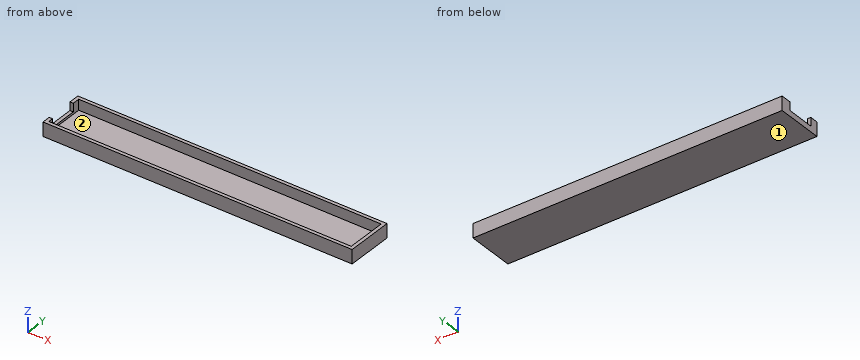
```python
from build123d import *

# Parameters (mm, degrees)
F0_W     = 110.8
F0_H     = 16.8
F0_W_2   = 110
F0_H_2   = 16
F1_DEPTH = 5
F2_T     = -1.2
F4_W     = 10
F4_H     = 3
F5_DEPTH = 2


with BuildPart() as f1:
    # F0 (on Top) → F1 (new body)
    with BuildSketch(Plane.XY):
        Rectangle(F0_W, F0_H)
        Rectangle(F0_W_2, F0_H_2, mode=Mode.SUBTRACT)
        Rectangle(F0_W_2, F0_H_2)
    extrude(amount=F1_DEPTH)

    # F2
    f2_openings = [f1.faces().sort_by_distance(p)[0] for p in [
        (0, 0, 5),
    ]]
    offset(amount=F2_T, openings=f2_openings)

    # F4 (on offset) → F5 (cut)
    with BuildSketch(Plane(origin=(-55.4, 0, 0), x_dir=(0, -1, 0), z_dir=(-1, 0, 0))):
        with Locations((0.4, 3.5)):
            Rectangle(F4_W, F4_H)
    extrude(amount=-F5_DEPTH, mode=Mode.SUBTRACT)


solid = f1.part
```
CAD build for the part. Positions are in the model's coordinates, mm. Face numbers are marked on the shaded views. Round coordinates to 2 decimals unless told otherwise and drop trailing zeros. Order: outer loops, then holes, each group sorted by start corner. A loop starts at its lowest first (then second) coordinate and runs counter-clockwise, first axis right, second up.
Item 1: Saw through at A-A on x = 31.5. Write the cut outline in (y, z).
Item 2: Saw through at C-C on z = 4.1. Write the cut outline in (x, y).
Item 3: Saw through at B-B on y = -4. Write the cut outline in (x, z).
Item 4: Pin check, flat tips, straight feed: pin 1 (4 mm diameter, centred on x = -13.5, y = 3, fed in from +Z); pin 2 (5 mm diameter, centred on x = -32, y = -2.5, fed in from -Z); pin 3 (1.3 mm diameter, centred on x = -55, y = 1.5, fed in from +Z). Stop position of each tip, or through.
Item 5: Probe line 1 along Y through (x, z) = (-16, 4.75); line 2 along X through (y, z) = (5, 2); line 3 along Z through (x, y) = (37, 0). List the from-to ranges inside material, lowest first.
Item 6: Mould opens along Z. For the marked faces 1 and 2 say: pulls with the +Z half, pulls with the -Z half, needs draft (parallel to the pull), parting line crosses it, or undercut.
Reported:
1. outline: (-8.4, 0) - (8.4, 0) - (8.4, 5) - (7.2, 5) - (7.2, 1.2) - (-7.2, 1.2) - (-7.2, 5) - (-8.4, 5) - close
2. outline: (-55.4, -8.4) - (55.4, -8.4) - (55.4, 8.4) - (-55.4, 8.4) - (-55.4, 4.6) - (-54.2, 4.6) - (-54.2, 7.2) - (54.2, 7.2) - (54.2, -7.2) - (-54.2, -7.2) - (-54.2, -5.4) - (-55.4, -5.4) - close
3. outline: (-55.4, 0) - (55.4, 0) - (55.4, 5) - (54.2, 5) - (54.2, 1.2) - (-54.2, 1.2) - (-54.2, 2) - (-55.4, 2) - close
4. pin 1: stops at z = 1.2
4. pin 2: stops at z = 0
4. pin 3: stops at z = 2
5. line 1: y = -8.4 to -7.2, 7.2 to 8.4
5. line 2: x = -55.4 to -54.2, 54.2 to 55.4
5. line 3: z = 0 to 1.2
6. face 1: pulls with the -Z half
6. face 2: pulls with the +Z half
